Source: three-view drawing plus pictorial views. Frame: mm from the lowest corner of the part. A direction names the side the tool comes from. Give positions to 0.01 mm unless a question says otherwise; leave off trailing zeros. Loops run counter-clockwise (first coordinate to the right, second up) from the corner with the lowest first, then second, coordinate; pieces in that order, holes last. Notation, with made-up numbers: (52.5, 79.25) -> (88.5, 79.25) arc R27 ccw to (88.5, 113.25) -> close; hole circle Ø5 at (-29.75, -24). An arc over 180 degrees is marked (long way). Answer in a Markdown table with one row per item. Add a question column.
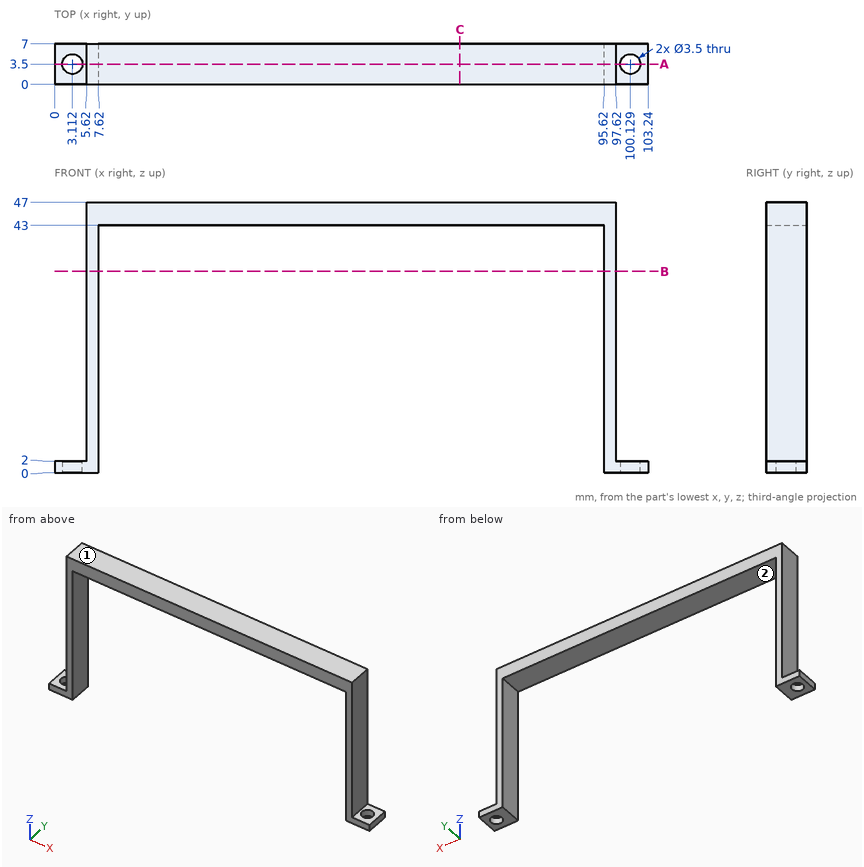
(1) Cut plane C-C on x = 70.5. Return the cut outline in (y, z), then the cut area to 3 significant figures.
(2) Cut plane B-B on z = 35. Return the cut outline in (x, y).
(3) Cut plane A-A on y = 3.5. Return the cut outline in (x, z).
(4) Reachability of the marked faces 1 and 2 from +Z, -Z, +X, -X, +Y, -Y: full face, straight path, thin tool, end or side. Return the list, or none.
(5) Material intervals for line 1 along X through (y, z) = (3, 37.5); line 2 along Z through (x, y) = (29.5, 4.75), sorted ascending. Write a range as from..to.
(6) Pin query (flat end, axial travel): pin 1 Ø1.7 at (x, y) = (2.5, 2.5) entering from +Z; pin 2 Ø4 at (x, y) = (46, 4.5) entering from -Z; pin 3 Ø2 at (x, z) = (10.5, 31.5) entering from -Y; pin 4 Ø3.5 at (y, z) = (3.5, 30) entering from -X. Return the tip coordinate at first contact, or that it passes through.
Answer list:
| question | item | result |
|---|---|---|
| 1 | outline | (0, 43) -> (7, 43) -> (7, 47) -> (0, 47) -> close |
| 1 | area | 28.0 mm² |
| 2 | outline | (5.62, 0) -> (7.62, 0) -> (7.62, 7) -> (5.62, 7) -> close; (95.62, 0) -> (97.62, 0) -> (97.62, 7) -> (95.62, 7) -> close |
| 3 | outline | (0, 0) -> (1.36, 0) -> (1.36, 2) -> (0, 2) -> close; (4.86, 0) -> (7.62, 0) -> (7.62, 43) -> (95.62, 43) -> (95.62, 0) -> (98.38, 0) -> (98.38, 2) -> (97.62, 2) -> (97.62, 47) -> (5.62, 47) -> (5.62, 2) -> (4.86, 2) -> close; (101.88, 0) -> (103.24, 0) -> (103.24, 2) -> (101.88, 2) -> close |
| 4 | face 1 | +Z, +X, -X, +Y, -Y |
| 4 | face 2 | -Z, +Y, -Y |
| 5 | line 1 | x = 5.62..7.62, 95.62..97.62 |
| 5 | line 2 | z = 43..47 |
| 6 | pin 1 | stops at z = 2 |
| 6 | pin 2 | stops at z = 43 |
| 6 | pin 3 | passes through |
| 6 | pin 4 | stops at x = 5.62 |
